Autodesk Inventor part; units mm, degrees
ref_plane "Work Plane2" through (0, 4, 0) normal (0, -1, 0) x (1, 0, 0)
ref_plane "Work Plane1" through (-24.5, 7, -5) normal (0, 1, 0) x (1, 0, 0)
ref_plane "YZ Plane" through (0, 0, 0) normal (1, 0, 0) x (0, 1, 0)
sketch "Sketch1" plane through (0, 0, 0) normal (0, 1, 0) x (-1, 0, 0)
  circle A0 centre (0, 0) radius 3.1
  circle A1 centre (49, 0) radius 3.1
  circle A2 centre (49, -58) radius 3.1
  circle A3 centre (0, -58) radius 3.1
  dimension "d4" = 6.2
  dimension "d5" = 6.2
  dimension "d6" = 6.2
  dimension "d7" = 6.2
  dimension "d12" = 58
  dimension "d13" = 58
  dimension "d14" = 49
  dimension "d15" = 49
extrude "Extrusion1" add sketch "Sketch1" along normal blind 2
sketch "Sketch3" plane through (0, 2, 0) normal (0, 1, 0) x (1, 0, 0)
  circle A0 centre (0, 0) radius 3.1
  circle A1 centre (0, 0) radius 3.625
  circle A2 centre (0, 58) radius 3.1
  circle A3 centre (0, 58) radius 3.625
  circle A4 centre (-49, 58) radius 3.1
  circle A5 centre (-49, 58) radius 3.625
  circle A6 centre (-49, 0) radius 3.1
  circle A7 centre (-49, 0) radius 3.625
  line L0 (-52.625, 0) -> (-52.625, 58)
  line L1 (-49, 61.625) -> (0, 61.625)
  line L2 (3.625, 58) -> (3.625, 0)
  line L3 (0, -3.625) -> (-49, -3.625)
  dimension "d18" = 7.25
  dimension "d19" = 7.25
  dimension "d20" = 7.25
  dimension "d21" = 7.25
extrude "Extrusion2" add sketch "Sketch3" along normal blind 2 contours A0 | A1 | A1 L3 A7 L0 A5 L1 A3 L2 | A3 | A7 | A5 | A2 | A4 | A6
sketch "Sketch5" plane through (0, 2, 0) normal (0, -1, 0) x (1, 0, 0)
  circle A0 centre (-4.375, -6.375) radius 4
  circle A1 centre (-44.625, -6.375) radius 4
  line L0 (3.625, 0) -> (3.625, -58)
  line L1 (-52.625, -58) -> (-52.625, 0)
  line L2 (-49, 3.625) -> (0, 3.625)
  line L3 (-4.375, -2.375) -> (-44.625, -2.375)
  line L4 (-4.375, -10.375) -> (-44.625, -10.375)
  circle A2 centre (-4.375, -17.625) radius 4
  line L5 (-4.375, -13.625) -> (-44.625, -13.625)
  line L6 (-4.375, -21.625) -> (-44.625, -21.625)
  circle A3 centre (-44.625, -17.625) radius 4
  circle A4 centre (-4.375, -28.875) radius 4
  line L7 (-4.375, -24.875) -> (-44.625, -24.875)
  line L8 (-4.375, -32.875) -> (-44.625, -32.875)
  circle A5 centre (-44.625, -28.875) radius 4
  circle A6 centre (-4.375, -40.125) radius 4
  line L9 (-4.375, -36.125) -> (-44.625, -36.125)
  line L10 (-4.375, -44.125) -> (-44.625, -44.125)
  circle A7 centre (-44.625, -40.125) radius 4
  circle A8 centre (-4.375, -51.375) radius 4
  line L11 (-4.375, -47.375) -> (-44.625, -47.375)
  line L12 (-4.375, -55.375) -> (-44.625, -55.375)
  circle A9 centre (-44.625, -51.375) radius 4
  point P0 (0, 0)
  dimension "d27" = 8
  dimension "d28" = 8
  dimension "d29" = 8
  dimension "d30" = 8
  dimension "d31" = 10
  dimension "d32" = 10
  dimension "d35" = 11.25
extrude "Extrusion3" cut sketch "Sketch5" against normal blind 2
sketch "Sketch6" plane through (0, 0, 0) normal (0, -1, 0) x (1, 0, 0)
  circle A0 centre (0, 0) radius 3.1
  circle A1 centre (-49, -58) radius 3.1
  line L0 (0, 0) -> (-49, 0)
  line L1 (-49, 0) -> (-49, -58)
  line L2 (-49, -58) -> (0, -58)
  line L3 (0, -58) -> (0, 0)
hole "Hole1" at (0, 0, -58) at (0, 0, 0) at (-49, 0, 0) at (-49, 0, -58) direction (0, 1, 0) diameter 2 end through all
sketch "Sketch7" plane through (0, 4, 0) normal (0, 1, 0) x (1, 0, 0)
  circle A0 centre (-24.5, 52.875) radius 4
  circle A1 centre (-24.5, 4.875) radius 4
  line L0 (-49, -3.625) -> (0, -3.625)
  point P0 (0, 0)
  dimension "d49" = 8
  dimension "d50" = 8
  dimension "d51" = 48
  dimension "d52" = 8.5
ref_plane "Work Plane2" through (0, 4, 0) normal (0, -1, 0) x (1, 0, 0)
sketch "Sketch8" plane through (0, 4, 0) normal (0, -1, 0) x (1, 0, 0)
  line L0 (-29.5, -61.5) -> (-19.5, -61.5)
  line L1 (-19.5, -61.5) -> (-19.5, 3.5)
  line L2 (-19.5, 3.5) -> (-29.5, 3.5)
  line L3 (-29.5, 3.5) -> (-29.5, -61.5)
  arc A0 (-27.6225, -2.5) -> (-21.3775, -2.5) centre (-24.5, -5) ccw
  point P0 (0, 0)
  dimension "d55" = 10
  dimension "d56" = 5
extrude "Extrusion5" add sketch "Sketch8" along normal up to surface (2 mm away)
ref_plane "Work Plane1" through (-24.5, 7, -5) normal (0, 1, 0) x (1, 0, 0)
extrude "Extrusion6" cut sketch "Sketch7" against normal blind 10
equation "\"d18\" = d19"
equation "\"d20\" = d19"
equation "\"d21\" = d19"
properties part number "Pi_mount"
Input: part model. Units: mm. Frame: model coordinates. A direction names the side the tool comes from. Give positions to 0.01 mm unless a question says otherwise; leave off trailing zeros. Order: outer loops, then holes, each group sorted by start corner. A loop starts at its lowest first (then second) coordinate and runs counter-clockwise, first axis right, second up. Notation, with made-up numbers: M 58,65.25 L 97,65.25 A15 ccw 97,75.25 Z; hole C 13,79.5 d3. An arc over 180 degrees is marked long. One line per question, with ' | ' between items.
1) Section D-D on z = -50. Output: boundary loops of the cut face in (x, y) (3 decimals).
Filled in:
outline: M -52.625,2 L -48.381,2 L -48.381,4 L -52.625,4 Z; M -29.5,2 L -27.281,2 L -27.281,4 L -29.5,4 Z; M -21.719,2 L -19.5,2 L -19.5,4 L -21.719,4 Z; M -0.619,2 L 3.625,2 L 3.625,4 L -0.619,4 Z
2) Section C-C on x = -9. Output: boundary loops of the cut face in (y, z) (3 decimals).
Filled in:
outline: M 2,-61.625 L 4,-61.625 L 4,-55.375 L 2,-55.375 Z; M 2,-47.375 L 4,-47.375 L 4,-44.125 L 2,-44.125 Z; M 2,-36.125 L 4,-36.125 L 4,-32.875 L 2,-32.875 Z; M 2,-24.875 L 4,-24.875 L 4,-21.625 L 2,-21.625 Z; M 2,-13.625 L 4,-13.625 L 4,-10.375 L 2,-10.375 Z; M 2,-2.375 L 4,-2.375 L 4,3.625 L 2,3.625 Z
3) Section A-A on y = 1.35. Output: boundary loops of the cut face in (x, z), and give its area (3 significant figures).
Filled in:
outline: C -49,-58 d6.2; C -49,0 d6.2; C 0,-58 d6.2; C 0,0 d6.2; hole C -49,-58 d2; hole C -49,0 d2; hole C 0,-58 d2; hole C 0,0 d2 | area: 108 mm2
4) Contact query for a flat-ended pin moving along its axis: P1, Ø2.5, axis at x = 0, z = 0, coming from the +Y side. Output: stop coordinate, or through.
Filled in:
P1: stops at y = 4
5) Access query for faces 4 (the face through (-25, 4, -29)), 5 (the face through (-19.5, 3, -18)), 6 (the face through (-25, 2, -29)). Directions: +Z, -Z, +X, -X, +Y, -Y. A direction counts if a zero-diameter tool reaches every point of the face in a straight line with its end or side. Return the directions, or none.
Filled in:
face 4: +Z, -Z, +X, -X, +Y | face 5: +Y, -Y | face 6: -Y
6) Draft query along Z for faces 1 (the face through (-51.535, 2.986, 2.591)), 2 (the face through (1, 0, 1)), 3 (the face through (-12, 3, -24.875)). Return one class per face: pulls with the +Z half, pulls with the -Z half, needs draft (parallel to the pull), parting line crosses it, or undercut.
Filled in:
face 1: pulls with the +Z half | face 2: needs draft | face 3: undercut
7) Ray query, L1, parallel to Z at x = -17, y = 2.25 (3 decimals); L2, parallel to Z at x = -49, y = 1.85; L3, parallel to Z at x = -24.5, y = 3.3 (3 decimals). Return the intervals inside material, ascending.
Filled in:
L1: z = -61.625 to -55.375, -47.375 to -44.125, -36.125 to -32.875, -24.875 to -21.625, -13.625 to -10.375, -2.375 to 3.625 | L2: z = -61.1 to -59, -57 to -54.9, -3.1 to -1, 1 to 3.1 | L3: z = -61.625 to -56.875, -48.875 to -8.875, -0.875 to 3.625
8) Section B-B on x = -24.5. Output: boundary loops of the cut face in (y, z) (3 decimals), and give its area (3 significant figures).
Filled in:
outline: M 2,-61.625 L 4,-61.625 L 4,-56.875 L 2,-56.875 Z; M 2,-48.875 L 4,-48.875 L 4,-8.875 L 2,-8.875 Z; M 2,-0.875 L 4,-0.875 L 4,3.625 L 2,3.625 Z | area: 98.5 mm2
